Work out the finished part from the listing and answer in its coordinate system (mm). Face numbers are marked on the shaded views. A direction names the side the tool comes from. Give positions to 0.01 mm unless a question says otherwise; leave off trailing zeros. Order: outer loops, then holes, each group sorted by start corner. A loop starts at its lowest first (then second) coordinate and runs counter-clockwise, first axis right, second up. Notation, with made-up numbers: (-5.5, 67.25) - (35.5, 67.25) arc R22 cw to (35.5, 94.25) - close; hole circle Ø3 at (62, -33.75). An arc over 180 degrees is marked (long way). Return JSON: item names as keys, results as strings. Group by question number.
from build123d import *

# Parameters (mm, degrees)
F1_DEPTH  = 5
F3_DEPTH  = 8
F4_R      = 2
F5_DEPTH  = 10
F6_R      = 2
F7_DEPTH  = 12
F7_TAPER  = 3
F8_R      = 2.9
F9_DEPTH  = 8
F18_DEPTH = 26


with BuildPart() as f1:
    # F0 (on Top) → F1 (new body)
    with BuildSketch(Plane.XY):
        with BuildLine():
            Line((6, -44), (6, 0))
            ThreePointArc((6, 0), (-4.582575695, 3.8729833462), (1, -5.9160797831))
            Line((1, -5.9160797831), (1, -39))
            Line((1, -39), (6, -44))
        make_face()
    extrude(amount=F1_DEPTH)

    # F2 (on face) → F3 (join)
    with BuildSketch(Plane.XY.offset(5)):
        with BuildLine():
            ThreePointArc((6, 0), (4.582575695, -3.8729833462), (1, -5.9160797831))
            Line((1, -5.9160797831), (1, -39))
            Line((1, -39), (6, -44))
            Line((6, -44), (6, 0))
        make_face()
    extrude(amount=F3_DEPTH)

    # F4 (on face) → F5 (cut)
    with BuildSketch(Plane.XY.offset(13)):
        with Locations((3.5, -10.9160797831)):
            Circle(F4_R)
    extrude(amount=-F5_DEPTH, mode=Mode.SUBTRACT)

    # F6 (on face) → F7 (join)
    with BuildSketch(Plane.XY.offset(13)):
        with Locations((3.5, -34.916)):
            Circle(F6_R)
    extrude(amount=F7_DEPTH, taper=F7_TAPER)

    # F8 (on face) → F9 (join, through all)
    with BuildSketch(Plane.XY.offset(5)):
        Circle(F8_R)
    extrude(amount=F9_DEPTH)


with BuildPart() as f10_1:
    # F10: instance of F1
    add(f1.part.mirror(Plane(origin=(3.6215352024, -22.9951774059, 13), x_dir=(1, 0, 0), z_dir=(0, 0, 1))))

    # F14: sweep along a path in F12
    with BuildLine(Plane(origin=(0, 0, 13), x_dir=(1, 0, 0), z_dir=(0, 0, -1))) as f14_path:
        Line((1, 29), (-4, 29))
        ThreePointArc((-4, 29), (-9, 24), (-4, 19))
    # F13 (on face) → F14 (sweep)
    with BuildSketch(Plane(origin=(1, 0, 0), x_dir=(0, -1, 0), z_dir=(-1, 0, 0))):
        with BuildLine():
            ThreePointArc((31.5, 13), (29, 15.5), (26.5, 13))
            Line((26.5, 13), (31.5, 13))
        make_face()
    sweep(path=f14_path.line)

    # F15 (on face) → F16 (revolve)
    with BuildSketch(Plane.YZ.offset(-4)):
        with BuildLine():
            Line((-19, 13), (-16.5, 13))
            ThreePointArc((-16.5, 13), (-17.232233047, 14.767766953), (-19, 15.5))
            Line((-19, 15.5), (-19, 13))
        make_face()
    revolve(axis=Axis((-4, -19, 14.25), (0, 0, 1)))

    # F17 (on face) → F18 (join)
    with BuildSketch(Plane.XY.offset(26)):
        with BuildLine():
            Line((-8.4852813742, -7.0710678119), (-7.7781745931, -7.7781745931))
            ThreePointArc((-7.7781745931, -7.7781745931), (-4.209517756, -10.1626748576), (0, -11))
            Line((0, -11), (1, -11))
            Line((1, -11), (1, -5.9160797831))
            ThreePointArc((1, -5.9160797831), (-2.2961005942, -5.5432771951), (-4.8904069139, -3.4761933515))
            Line((-4.8904069139, -3.4761933515), (-8.4852813742, -7.0710678119))
        make_face()
    extrude(amount=-F18_DEPTH)


solid = f10_1.part
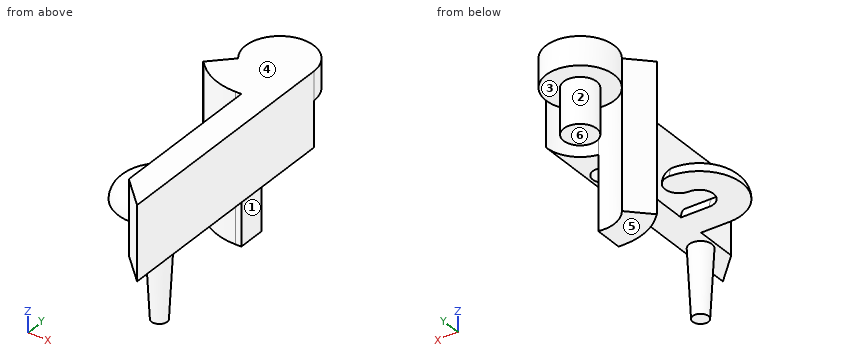
1. Each of these flat-tipped pins is pushed along its axis until it touches: pin 1 (5.5 mm diameter, centred on y = -8, z = 4, fed in from +X); pin 2 (2 mm diameter, centred on x = 4, y = -35.5, fed in from -Z); pin 3 (1.1 mm diameter, centred on x = 0.5, z = 6.5, fed in from -Y); pin 4 (2 mm diameter, centred on x = -7.5, y = -11.5, fed in from +Z). Where does it stop, or does it pass through?
2. The part is cut by section A-A (z = 4.75). Give the vertices of the cut face in (x, y).
3. A tool of negligible diameter and unlimited length cuts with its end or side. For the marked faces 5 and 6, from which of +Z, -Z, +X, -X, +Y, -Y can it reach the whole face along a straight path? Write none if from no direction.
4. The part is cut by section C-C (x = -2.25). Give the vertices of the cut face in (y, z).
5. The part is cut by section D-D (z = 21.75). Give the vertices of the cut face in (x, y).
6. Determine the mould class of the marked faces 1, 2, 3 and 4 for opening direction X: released by +X, released by -X, zero draft, split by the parting line, or undercut.
7. Consider probe 1 along Z at (x, y) = (3.75, -11.5); probe 2 along Z at (x, y) = (5, -17.5); probe 3 along X at (y, z) = (-5, 17.5). Determine where each line is inside the solid, lowest interval first. Write a range as from..to.
8. The part is cut by section B-B (z = 14). Give the vertices of the cut face in (x, y).
Answers:
{
 "1": {"pin 1": "stops at x = 1", "pin 2": "stops at z = 1", "pin 3": "stops at y = -11", "pin 4": "passes through"},
 "2": {"outline": "(-8.49, -7.07) - (-7.78, -7.78) arc R11 ccw to (0, -11) - (1, -11) - (1, -5.92) arc R6 cw to (-4.89, -3.48) - close; circle Ø3.14 at (3.5, -34.92)"},
 "3": {"face 5": "-Z, +X, -X, +Y, -Y", "face 6": "-Z, +X, -X, +Y"},
 "4": {"outline": "(-31.5, 13) - (-26.5, 13) arc R2.5 ccw to start; (-20.79, 13) - (-17.21, 13) arc R1.79 ccw to start; (-10.77, 0) - (-5.56, 0) - (-5.56, 21) - (-1.83, 21) - (-1.83, 13) - (1.83, 13) - (1.83, 21) - (5.56, 21) - (5.56, 26) - (-10.77, 26) - close"},
 "5": {"outline": "(-8.49, -7.07) - (-7.78, -7.78) arc R11 ccw to (0, -11) - (1, -11) - (1, -39) - (6, -44) - (6, 0) arc R6 ccw (long way) to (-4.89, -3.48) - close; hole circle Ø4 at (3.5, -10.92)"},
 "6": {"face 1": "released by +X", "face 2": "undercut", "face 3": "undercut", "face 4": "zero draft"},
 "7": {"probe 1": "z = 23..26", "probe 2": "z = 13..26", "probe 3": "x = -6.41..-3.32, 3.32..6"},
 "8": {"outline": "(-8.49, -7.07) - (-7.78, -7.78) arc R11 ccw to (0, -11) - (1, -11) - (1, -26.71) - (-4, -26.71) arc R2.71 cw to (-4, -21.29) arc R2.29 ccw to (-4, -16.71) arc R7.29 ccw to (-4, -31.29) - (1, -31.29) - (1, -39) - (6, -44) - (6, 0) arc R6 cw to (-4.89, -3.48) - close; circle Ø5.8 at (0, 0); hole circle Ø4 at (3.5, -10.92)"}
}
